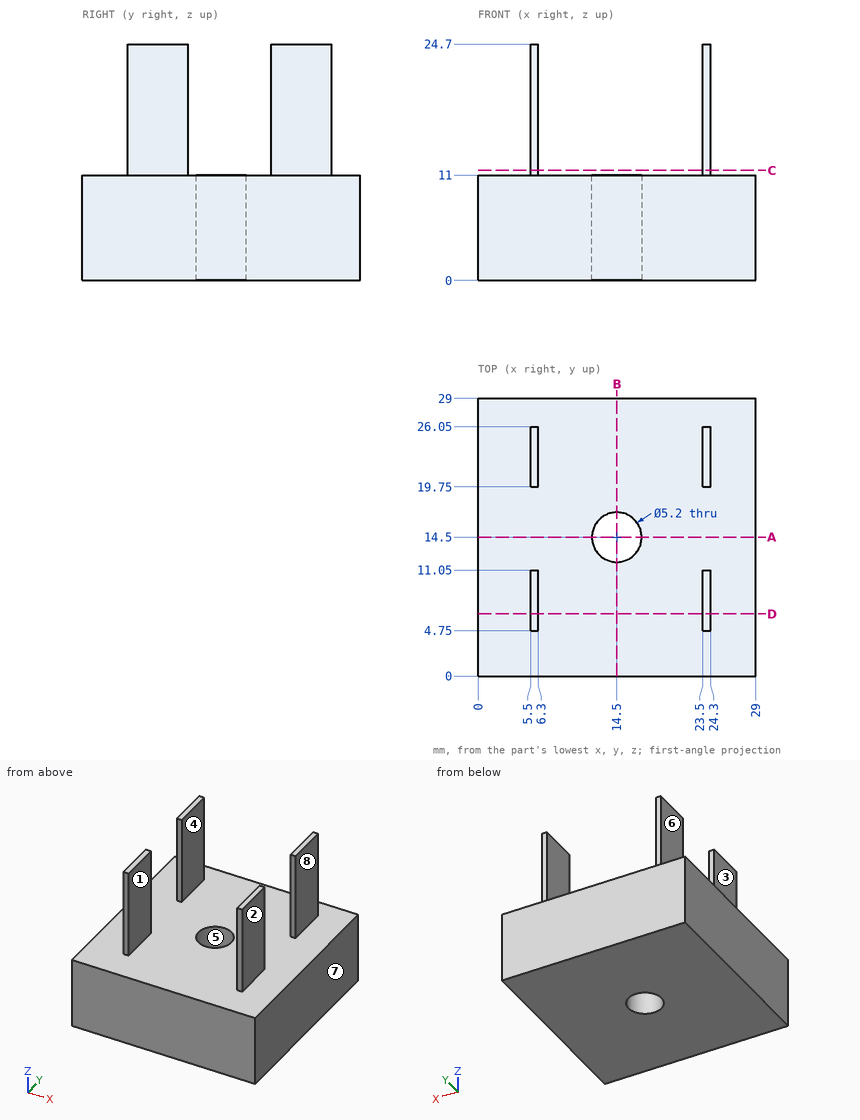
Drawing for the job (mm, zero at the part's lowest x, y, z). A direction names the side the tool comes from. Coordinates: 2 decimals unless noted, no trailing zeros. Order: outer loops, then holes, each group sorted by start corner. A loop starts at its lowest first (then second) coordinate and runs counter-clockwise, first axis right, second up. Notation, with made-up numbers: (37, 70) -> (69, 70) arc R6 cw to (69, 74) -> close; hole circle Ø5 at (-35.5, -33.5). An arc over 180 degrees is marked (long way). Answer in a Markdown table with one row per item.
1) Drill centre lines: line 1 (X direction, y = 24, z = 15.75); line 2 (Y direction, x = 14.5, z = 6); line 3 (Z direction, x = 20.75, y = 24.75). Where is each one in solid material? Low to high.
Check values:
| item | result |
|---|---|
| line 1 | 5.5 to 6.3, 23.5 to 24.3 |
| line 2 | 0 to 11.9, 17.1 to 29 |
| line 3 | 0 to 11 |
2) Which spindle directions (+Z, -Z, +X, -X, +Y, -Y) get a long thin tool onto all of the face, cutting with end or side? Do the marked faces 4, 5, 6, 7 and 8. Say none if no direction does.
Check values:
| item | result |
|---|---|
| face 4 | +Z, +Y, -Y |
| face 5 | +Z, -Z |
| face 6 | +Z, -X, +Y, -Y |
| face 7 | +Z, -Z, +X, +Y, -Y |
| face 8 | +Z, +X, +Y, -Y |
3) Mould opens along X. For the marked faces 1, 2 and 3 say: pulls with the +X half, pulls with the -X half, needs draft (parallel to the pull), parting line crosses it, or undercut.
Check values:
| item | result |
|---|---|
| face 1 | undercut |
| face 2 | pulls with the +X half |
| face 3 | pulls with the -X half |
4) Flat gauge pins, fed straight in: P1, Ø0.6, axis at x = 6, z = 19.5, coming from the +Y side; P2, Ø5, axis at x = 17, y = 22.5, coming from the +Z side; P3, Ø5, axis at y = 24, z = 19, coming from the +X side. Where does each tip first touch, or does it go through?
Check values:
| item | result |
|---|---|
| P1 | y = 26.05 |
| P2 | z = 11 |
| P3 | x = 24.3 |
5) Band-saw the part on C-C (z = 11.5). List the corners of the cut face in (x, y), and give its area (3 significant figures).
Check values:
| item | result |
|---|---|
| outline | (5.5, 4.75) -> (6.3, 4.75) -> (6.3, 11.05) -> (5.5, 11.05) -> close; (5.5, 19.75) -> (6.3, 19.75) -> (6.3, 26.05) -> (5.5, 26.05) -> close; (23.5, 4.75) -> (24.3, 4.75) -> (24.3, 11.05) -> (23.5, 11.05) -> close; (23.5, 19.75) -> (24.3, 19.75) -> (24.3, 26.05) -> (23.5, 26.05) -> close |
| area | 20.2 mm2 |
6) Band-saw the part on A-A (y = 14.5). List the corners of the cut face in (x, z), and give its area (3 significant figures).
Check values:
| item | result |
|---|---|
| outline | (0, 0) -> (11.9, 0) -> (11.9, 11) -> (0, 11) -> close; (17.1, 0) -> (29, 0) -> (29, 11) -> (17.1, 11) -> close |
| area | 262 mm2 |
7) Band-saw the part on D-D (y = 6.5). List the corners of the cut face in (x, z), and give its area (3 significant figures).
Check values:
| item | result |
|---|---|
| outline | (0, 0) -> (29, 0) -> (29, 11) -> (24.3, 11) -> (24.3, 24.7) -> (23.5, 24.7) -> (23.5, 11) -> (6.3, 11) -> (6.3, 24.7) -> (5.5, 24.7) -> (5.5, 11) -> (0, 11) -> close |
| area | 341 mm2 |
